Could you check a few things on this model? Use its own coordinates, in mm. Face numbers are marked on the shaded views. A direction names the side the tool comes from. Coordinates: 2 decimals unless noted, no trailing zeros. Loops run counter-clockwise (first coordinate to the right, second up) from the corner with the lowest first, then second, coordinate; pieces in that order, holes last. Notation, with made-up numbers: (-23.75, 75) -> (5.25, 75) arc R3 cw to (5.25, 79) -> close; hole circle Ø9 at (43, 56). An arc over 180 degrees is marked (long way). One line per question, with ' | ' between items.
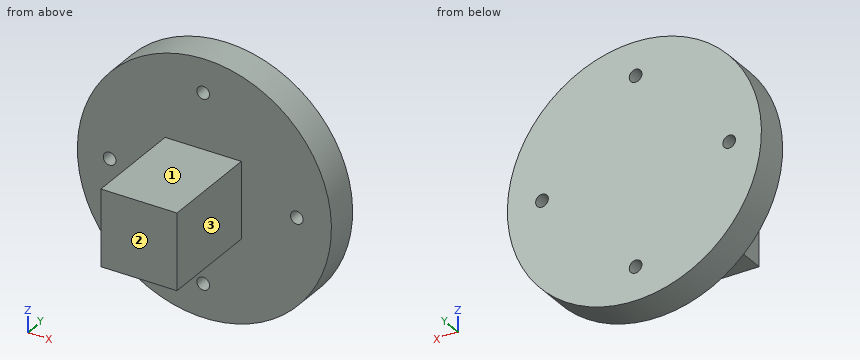
from build123d import *

# Parameters (mm, degrees)
SKETCH1_W           = 18
SKETCH1_H           = 18
BOSS_EXTRUDE1_DEPTH = 24.25
SKETCH2_R           = 30
BOSS_EXTRUDE2_DEPTH = 8
SKETCH3_R           = 1.5
CUT_EXTRUDE1_DEPTH  = 12


with BuildPart() as part:
    # Sketch1 → Boss-Extrude1 (new body)
    with BuildSketch(Plane(origin=(0, 0, 0), x_dir=(1, 0, 0), z_dir=(0, 1, 0))):
        Rectangle(SKETCH1_W, SKETCH1_H)
    extrude(amount=BOSS_EXTRUDE1_DEPTH)

    # Sketch2 → Boss-Extrude2 (add)
    with BuildSketch(Plane(origin=(0, 24.25, 0), x_dir=(1, 0, 0), z_dir=(0, 1, 0))):
        with Locations(Location((0.279992144, 0, 0), (0, 0, 270))):
            Circle(SKETCH2_R)
    extrude(amount=BOSS_EXTRUDE2_DEPTH)

    # Sketch3 → Cut-Extrude1 (cut)
    with BuildSketch(Plane(origin=(0, 32.25, 0), x_dir=(1, 0, 0), z_dir=(0, 1, 0))):
        with Locations(Location((0, 22.106714755, 0), (0, 0, 270))):
            Circle(SKETCH3_R)
        with Locations(Location((22.106714755, 0, 0), (0, 0, 270))):
            Circle(SKETCH3_R)
        with Locations(Location((0, -22.106714755, 0), (0, 0, 270))):
            Circle(SKETCH3_R)
        with Locations(Location((-22.106714755, 0, 0), (0, 0, 270))):
            Circle(SKETCH3_R)
    extrude(amount=-CUT_EXTRUDE1_DEPTH, mode=Mode.SUBTRACT)


solid = part.part
1) I need wall thicknesses on line 1 along X through (y, z) = (28, 0); line 2 along Y through (x, z) = (26, -4); line 3 along X through (y, z) = (18, 1.5). Which ranges of each line are inside material? Lowest first, please. Write a range as from..to.
Data:
line 1: -29.72..-23.61, -20.61..20.61, 23.61..30.28 | line 2: 24.25..32.25 | line 3: -9..9
2) If we section it at A-A on z = 0: Please give me the cut outline in (x, y).
Data:
outline: (-29.72, 24.25) -> (-23.61, 24.25) -> (-23.61, 32.25) -> (-29.72, 32.25) -> close; (-20.61, 24.25) -> (-9, 24.25) -> (-9, 0) -> (9, 0) -> (9, 24.25) -> (20.61, 24.25) -> (20.61, 32.25) -> (-20.61, 32.25) -> close; (23.61, 24.25) -> (30.28, 24.25) -> (30.28, 32.25) -> (23.61, 32.25) -> close
3) If we section it at D-D on z = -6: Please give me the cut outline in (x, y).
Data:
outline: (-29.11, 24.25) -> (-9, 24.25) -> (-9, 0) -> (9, 0) -> (9, 24.25) -> (29.67, 24.25) -> (29.67, 32.25) -> (-29.11, 32.25) -> close
4) I'm going to push flat-ended pins straight in: pin 1 Ø2 at (x, y) = (-8.5, 9) entering from -Z; pin 2 Ø6 at (y, z) = (21, -9) entering from -X; pin 3 Ø9 at (x, y) = (-0.5, 10.5) entering from +Z. Where does each tip first touch, or does it pass through?
Data:
pin 1: z = -9 | pin 2: x = -9 | pin 3: z = 9
5) If we section it at B-B on x = 3: Please give me the cut outline in (y, z).
Data:
outline: (0, -9) -> (24.25, -9) -> (24.25, -29.88) -> (32.25, -29.88) -> (32.25, 29.88) -> (24.25, 29.88) -> (24.25, 9) -> (0, 9) -> close
6) On a 3-axis mill with a long thin cutter (end or side, diameter ignored), from which of +Z, -Z, +X, -X, +Y, -Y can I reach the whole of each face in a straight line? I mean the marked faces 1, 2 and 3. Say none if no direction works.
Data:
face 1: +Z, +X, -X, -Y | face 2: +Z, -Z, +X, -X, -Y | face 3: +Z, -Z, +X, -Y
7) If we section it at C-C on y = 30: Please give me the cut outline in (x, z), and give its area (3 significant figures).
Data:
outline: circle Ø60 at (0.28, 0); hole circle Ø3 at (-22.11, 0); hole circle Ø3 at (0, -22.11); hole circle Ø3 at (0, 22.11); hole circle Ø3 at (22.11, 0) | area: 2,800 mm²
